Design review of the part built by this model. Coordinates are the model's own, in mm. A direction names the side the tool comes from. Coordinates: 2 decimals unless noted, no trailing zeros. Order: outer loops, then holes, each group sorted by start corner. A loop starts at its lowest first (then second) coordinate and runs counter-clockwise, first axis right, second up. Notation, with made-up numbers: (9, 54.5) -> (55, 54.5) arc R8 ccw to (55, 63.5) -> close; hole circle Ø1 at (47.25, 80). An arc over 180 degrees is marked (long way). Use a Markdown table: item, result. Add a question column.
Q1. Machinability: for faces 5 (the face through (-15.07, 10.95, 44.24)), 6 (the face through (0, 13, 20)), 7 (the face through (16, -7, 36.725)), which of the approach directions +Z, -Z, +X, -X, +Y, -Y give a long, thin tool a straight path to every point of the face, cutting with its end or side? Answer none if there is none.
Q2. The part is to be moulded in two halves that separate along Y. For faces 1 (the face through (-18, 4, 43.275)), 2 (the face through (0.653, 20.264, 24.225)), 3 (the face through (-18.337, -3.274, 40.072)), 4 (the face through (0.05, -12.59, 12.37)), say which applies: pulls with the +Y half, pulls with the -Y half, needs draft (parallel to the pull), parting line crosses it, or undercut.
Q3. Add section C-C (z = -7). State the section outline as (x, y) points.
Q4. Wall thickness on probe 1 along Y at (x, z) = (0, -10.5); probe 2 along X at (y, z) = (0, 33) (3 decimals); probe 3 along Y at (x, z) = (0, 2) (3 decimals): over which ranges is each line inside the solid? List them lowest first.
Q5. Add section B-B (x = 0). State the section outline as (y, z) points (3 decimals).
Q6. Add section D-D (z = 21.5). State the section outline as (x, y) points (3 decimals), then the cut area to 3 significant figures.
Q7. Insertion check: pin 1 (1.2 mm diameter, centred on y = -12.5, z = 15.5, fed in from +X); pin 2 (5 mm diameter, centred on x = -11.5, z = 36, fed in from -Y); pin 3 (1 mm diameter, centred on x = 16, z = 3.5, fed in from +Y). Each pin has a flat end and moves straight along its axis. Give the tip position at first contact, or say it passes through.
from build123d import *

# Parameters (mm, degrees)
F2_R          = 3.275
F3_DEPTH      = 25
F4_W          = 4
F4_H          = 6.55
F5_ANGLE      = 60
F6_W          = 4
F6_H          = 6.55
F7_ANGLE      = 60
F9_DEPTH      = 10
F10_W         = 32
F10_H         = 8
F11_DEPTH     = 50.0010001
F12_W         = 7
F12_H         = 7
F13_DEPTH     = 5
F15_DEPTH     = 3.5
F16_R         = 2
F17_R         = 3.4
F18_R         = 16.5
F18_R_2       = 12.5
F19_DEPTH     = 25
F20_T4_ANGLE  = 270.7214927844
F20_S5_R      = 20.275
F20_T6_DEPTH  = 31
F20_T11_ANGLE = 90.6289211612
F20_S12_R     = 20.275
F20_T13_DEPTH = 16
F21_T4_DEPTH  = 44.6904958407
F21_S5_R      = 16.5
F21_T6_DEPTH  = 24


# Not quite as in the source:
# - a fillet or chamfer that OpenCascade refuses, or shapes differently, is made with other operations: its cross-section is extruded or revolved along the edge and cut away or added


with BuildPart() as f1:
    # F0 (on Front) → F1 (revolve)
    with BuildSketch(Plane.XZ):
        Polygon((20.275, 50), (16.775, 50), (16.775, 20), (12.5, 20), (12.5, 0), (20.275, 0), align=None)
    revolve(axis=Axis((0, 0, 24.5366517103), (0, 0, 1)))

    # F2 (on Right) → F3 (cut, symmetric)
    with BuildSketch(Plane.YZ):
        with Locations((0, 40)):
            Circle(F2_R)
    extrude(amount=F3_DEPTH, both=True, mode=Mode.SUBTRACT)

    # F4 (on Front) → F5 (revolve, cut)
    with BuildSketch(Plane.XZ):
        with Locations((18.275, 40)):
            Rectangle(F4_W, F4_H)
    revolve(axis=Axis((0, 0, 25.1644738019), (0, 0, -1)), revolution_arc=F5_ANGLE, mode=Mode.SUBTRACT)

    # F6 (on Front) → F7 (revolve, cut)
    with BuildSketch(Plane.XZ):
        with Locations((-18.275, 40)):
            Rectangle(F6_W, F6_H)
    revolve(axis=Axis((0, 0, 23.5361852683), (0, 0, -1)), revolution_arc=F7_ANGLE, mode=Mode.SUBTRACT)

    # F8 (on face) → F9 (cut)
    with BuildSketch(Plane.XY.offset(50)):
        with BuildLine():
            Line((-8.3875, 14.5275761485), (-10.1375, 17.5586650617))
            ThreePointArc((-10.1375, 17.5586650617), (-12.8757169507, 15.6617859137), (-15.2663853672, 13.342155104))
            Line((-15.2663853672, 13.342155104), (-13.3941586478, 10.0993633026))
            ThreePointArc((-13.3941586478, 10.0993633026), (-11.1136146512, 12.5653569144), (-8.3875, 14.5275761485))
        make_face()
        with BuildLine():
            Line((8.3875, -14.5275761485), (10.1375, -17.5586650617))
            ThreePointArc((10.1375, -17.5586650617), (12.8757169507, -15.6617859137), (15.2663853672, -13.342155104))
            Line((15.2663853672, -13.342155104), (13.3941586478, -10.0993633026))
            ThreePointArc((13.3941586478, -10.0993633026), (11.1136146512, -12.5653569144), (8.3875, -14.5275761485))
        make_face()
    extrude(amount=-F9_DEPTH, mode=Mode.SUBTRACT)

    # F10 (on face) → F11 (cut, through all)
    with BuildSketch(Plane.XY.offset(50)):
        with Locations((0, -17.5)):
            Rectangle(F10_W, F10_H)
    extrude(amount=-F11_DEPTH, mode=Mode.SUBTRACT)

    # F12 (on face) → F13 (cut)
    with BuildSketch(Plane.XZ.offset(13.5)):
        with Locations((0, 16.5)):
            Rectangle(F12_W, F12_H)
    extrude(amount=-F13_DEPTH, mode=Mode.SUBTRACT)

    # F14 (on Right) → F15 (cut, symmetric)
    with BuildSketch(Plane.YZ):
        Polygon((-10.3, 13), (-12.7, 13), (-11.2893841543, 5), (-10.3, 5), align=None)
    extrude(amount=F15_DEPTH, both=True, mode=Mode.SUBTRACT)

    # F16
    f16_edges = [f1.edges().sort_by_distance(p)[0] for p in [
        (15.661786, 12.875717, 50),
        (-20.274727, -0.105295, 50),
    ]]
    fillet(f16_edges, radius=F16_R)

    # F17
    f17_edges = [f1.edges().sort_by_distance(p)[0] for p in [
        (-14.330272, 11.720759, 43.275),
        (14.330272, -11.720759, 43.275),
    ]]
    fillet(f17_edges, radius=F17_R)

    # F18 (on face) → F19 (join)
    with BuildSketch(Plane(origin=(0, 0, 0), x_dir=(1, 0, 0), z_dir=(0, 0, -1))):
        Circle(F18_R)
        Circle(F18_R_2, mode=Mode.SUBTRACT)
    extrude(amount=F19_DEPTH)

    # F20: chamfer of 4 on 2 edges, made by hand


with BuildPart() as f20_tool2:
    # F20_s3 → F20_t4 (revolve)
    with BuildSketch(Plane(origin=(0, 0, 0), x_dir=(0, 0, 1), z_dir=(0.9999207165, 0.0125920918, 0))):
        Polygon((0, 20.5), (-4, 16.5), (0, 16.5), align=None)
    revolve(axis=Axis((0, 0, 0), (0, 0, -1)), revolution_arc=F20_T4_ANGLE)

    # F20_s5 → F20_t6 (intersect, symmetric)
    with BuildSketch(Plane.XY.offset(-2)):
        Circle(F20_S5_R)
    extrude(amount=F20_T6_DEPTH, both=True, mode=Mode.INTERSECT)

    split(bisect_by=Plane.XZ.offset(13.5), keep=Keep.BOTTOM)


with BuildPart() as f1_1:
    add(f1.part)

    # F20_t1: union F20_tool2
    add(f20_tool2.part)


with BuildPart() as f20_tool9:
    # F20_s10 → F20_t11 (revolve)
    with BuildSketch(Plane.XZ):
        Polygon((20.5, 0), (16.5, -4), (16.5, 0), align=None)
    revolve(axis=Axis((0, 0, 0), (0, 0, -1)), revolution_arc=F20_T11_ANGLE)

    # F20_s12 → F20_t13 (intersect, symmetric)
    with BuildSketch(Plane.XY.offset(-2)):
        Circle(F20_S12_R)
    extrude(amount=F20_T13_DEPTH, both=True, mode=Mode.INTERSECT)

    split(bisect_by=Plane.XZ.offset(13.5), keep=Keep.BOTTOM)


with BuildPart() as f1_2:
    add(f1_1.part)

    # F20_t8: union F20_tool9
    add(f20_tool9.part)

    # F21: chamfer of 5 on 1 edges, made by hand


with BuildPart() as f21_tool2:
    # F21_s3 → F21_t4 (new body)
    with BuildSketch(Plane.YZ.offset(-22.3452479203)):
        Polygon((-18.5, 0), (-13.5, 5), (-13.5, 0), align=None)
    extrude(amount=F21_T4_DEPTH)

    # F21_s5 → F21_t6 (intersect, symmetric)
    with BuildSketch(Plane.XY.offset(2.5)):
        Circle(F21_S5_R)
    extrude(amount=F21_T6_DEPTH, both=True, mode=Mode.INTERSECT)


with BuildPart() as f1_3:
    add(f1_2.part)

    # F21_t1: union F21_tool2
    add(f21_tool2.part)


solid = f1_3.part
Established:
| question | item | result |
|---|---|---|
| 1 | face 5 | +Y |
| 1 | face 6 | +Z |
| 1 | face 7 | +X, -Y |
| 2 | face 1 | needs draft |
| 2 | face 2 | parting line crosses it |
| 2 | face 3 | pulls with the +Y half |
| 2 | face 4 | undercut |
| 3 | outline | circle Ø33 at (0, 0); hole circle Ø25 at (0, 0) |
| 4 | probe 1 | -16.5 to -12.5, 12.5 to 16.5 |
| 4 | probe 2 | -20.275 to -16.775, 16.775 to 20.275 |
| 4 | probe 3 | -16.5 to -12.5, 12.5 to 20.275 |
| 5 | outline | (-16.5, -25) -> (-12.5, -25) -> (-12.5, 11.866) -> (-12.7, 13) -> (-13.5, 13) -> (-13.5, 5) -> (-16.5, 2) -> close; (12.5, -25) -> (16.5, -25) -> (16.5, -4) -> (20.275, -0.225) -> (20.275, 48) arc R2 ccw to (18.275, 50) -> (16.775, 50) -> (16.775, 20) -> (12.5, 20) -> close |
| 6 | outline | (-15.127, -13.5) -> (-9.957, -13.5) arc R16.775 cw (long way) to (9.957, -13.5) -> (15.127, -13.5) arc R20.275 ccw (long way) to start |
| 6 | area | 310 mm^2 |
| 7 | pin 1 | x = 16.42 |
| 7 | pin 2 | y = -13.5 |
| 7 | pin 3 | y = 13.07 |
